Source: CAD feature listing. Evaluate the final solid. Frame: model axes, mm. Round coordinates to 2 decimals unless told otherwise and drop trailing zeros. Write each loop counter-clockwise with the first axis right and the second up, starting at its lowest first coordinate (ties: lowest second). Pieces come first, ordered by that corner, then holes. Notation, with made-up numbers: (-26.5, 21) -> (21.5, 21) arc R18 ccw to (21.5, 40) -> close; hole circle Ø5 at (46, 7). An arc over 180 degrees is marked (long way). Return JSON: item names as keys, results as strings. Group by question number.
from build123d import *

# Parameters (mm, degrees)
F1_DEPTH = 1.5875
F2_R     = 19.04999
F3_R     = 6.35
F4_R     = 15.875
F5_DEPTH = 25.4


# Not quite as in the source:
# - a fillet or chamfer is up to 0.001 mm smaller than in the source, because OpenCascade refuses the exact size


with BuildPart() as f1:
    # F0 (on Right) → F1 (new body)
    with BuildSketch(Plane.YZ):
        Polygon((-77.51046875, 16.5875132085), (81.23953125, 16.5875132085), (81.23953125, -1.3419014323), (87.58953125, -1.3419014323), (87.58953125, 29.2875132085), (-39.41046875, 29.2875132085), (-39.41046875, 54.6875132085), (-77.51046875, 54.6875132085), align=None)
    extrude(amount=F1_DEPTH)

    # F2 (radius 19.05 in the source; OpenCascade refuses exactly that, so slightly less here)
    f2_edges = [f1.edges().sort_by_distance(p)[0] for p in [
        (0.79375, -77.510469, 54.687513),
        (0.79375, -77.510469, 16.587513),
        (0.79375, -39.410469, 54.687513),
    ]]
    fillet(f2_edges, radius=F2_R)

    # F3
    f3_edges = [f1.edges().sort_by_distance(p)[0] for p in [
        (0.79375, -39.410469, 29.287513),
    ]]
    fillet(f3_edges, radius=F3_R)

    # F4 (on face) → F5 (cut)
    with BuildSketch(Plane.YZ.offset(1.5875)):
        with Locations((-58.46046875, 35.6375132085)):
            Circle(F4_R)
    extrude(amount=-F5_DEPTH, mode=Mode.SUBTRACT)


solid = f1.part
Item 1: Cut plane C-C on z = 50. Output: boundary loops of the cut face in (x, y), and give its area (3 significant figures).
Item 2: Cut plane A-A on z = 39. Output: boundary loops of the cut face in (x, y), and give its area (3 significant figures).
Item 3: Material intervals for probe 1 along Y at (x, z) = (0.85, 35); probe 2 along Z at (x, y) = (1.3, -58); probe 3 along Z at (x, y) = (0.25, 61), sorted ascending.
Item 4: Pull-direction query (Z, two-part tool) for faces 1 (the cylindrical face through (0.8, -71.78, 22.02)), 2 (the cylindrical face through (0.805, -71.782, 49.255)), 3 (the cylindrical face through (0.8, -74.32, 36.34)), 4 (the flat face through (0, 11, 27)); classes: +Z half, -Z half, draft (parallel to the pull), parting line (faces both ways), or undercut.
Item 5: First-contact query: pin 1 Ø19 at (y, z) = (-58.46, 35.64) entering from +X; pin 2 Ø0.8 at (x, y) = (1, 44) entering from +Z. Flat tips, straight axial feed; report the tip coordinate or a pass-through.
Item 6: Cut plane D-D on y = 13. Output: boundary loops of the cut face in (x, z).
Here are the results:
{
 "1": {"outline": "(0, -70.98) -> (1.59, -70.98) -> (1.59, -65.22) -> (0, -65.22) -> close; (0, -51.7) -> (1.59, -51.7) -> (1.59, -45.95) -> (0, -45.95) -> close", "area": "18.3 mm^2"},
 "2": {"outline": "(0, -77.21) -> (1.59, -77.21) -> (1.59, -73.98) -> (0, -73.98) -> close; (0, -42.95) -> (1.59, -42.95) -> (1.59, -39.71) -> (0, -39.71) -> close", "area": "10.3 mm^2"},
 "3": {"probe 1": "y = -77.5 to -74.32, -42.6 to -39.38", "probe 2": "z = 16.59 to 19.77, 51.51 to 54.68", "probe 3": "z = 16.59 to 29.29"},
 "4": {"face 1": "-Z half", "face 2": "+Z half", "face 3": "undercut", "face 4": "draft"},
 "5": {"pin 1": "passes through", "pin 2": "stops at z = 29.29"},
 "6": {"outline": "(0, 16.59) -> (1.59, 16.59) -> (1.59, 29.29) -> (0, 29.29) -> close"}
}
